Build history of the part. All positions in model axes, mm. A direction names the side the tool comes from. Coordinates: 2 decimals unless noted, no trailing zeros. Loops run counter-clockwise (first coordinate to the right, second up) from the corner with the lowest first, then second, coordinate; pieces in that order, holes last.
(1) Slice it at B-B (z = 6). Give the number of separate pieces and of enclosed holes in the cut face, and give its area (3 significant figures).
(2) Two-plate mould, pull along Y, no slides. Class faces 1 (the face through (229.026, 329.954, 5.916)), 2 (the face through (229.853, 271.613, 5.916)), 3 (the face through (308, 350.56, 6)): pulls with the +Y half, pulls with the -Y half, needs draft (parallel to the pull), parting line crosses it, or undercut.
(3) Slice it at C-C (y = 346). Give the cut face in (x, z).
(4) Wall check: L1, parallel to Y at x = 250, z = 5; L2, parallel to X at y = 274.5, z = 10.5; L3, parallel to X at y = 303, z = 4.5. Give the ranges that are in metal, low to high.
(5) Flat gauge pins, fed straight in: P1, Ø1.5, axis at y = 254.5, z = 5, coming from the +X side; P2, Ø3, axis at y = 349, z = 5.5, coming from the +X side; P3, Ø0.8, axis at y = 348.5, z = 7.5, coming from the -X side; P4, Ø2.5, axis at x = 272.26, y = 244.39, coming from the +Z side. Where does each tip first touch, or does it go through?
(6) Slice it at D-D (x = 326). Give the cut face in (y, z), and give its area (3 significant figures).
(7) Slice it at A-A (x = 308). Give the cut face in (y, z), and give its area (3 significant figures).
(8) Tool access for faces 4 (the face through (309.564, 250.121, 5.916)), 5 (the face through (280, 357.622, 6)): list every direction of +Z, -Z, +X, -X, +Y, -Y with a clear straight run to the whole face (end or side of a thin tool).
from build123d import *

# Parameters (mm, degrees)
ESBO_O1_R                = 2
ESBO_O1_R_2              = 1.5
ESBO_O1_R_3              = 1
ESBO_O1_R_4              = 12
ESBO_O1_W                = 12
ESBO_O1_H                = 2.6
RESSALTO_EXTRUS_O1_DEPTH = 12


with BuildPart() as part:
    # Esboço1 → Ressalto-extrusão1 (new body)
    with BuildSketch(Plane.XY):
        Polygon((312.401923789, 240.878221735), (347.401923789, 301.5), (315, 357.621778265), (245, 357.621778265), (212.598076211, 301.5), (247.598076211, 240.878221735), align=None)
        with Locations((280, 253.378221735)):
            Circle(ESBO_O1_R, mode=Mode.SUBTRACT)
        with Locations((272.260343171, 244.388972359)):
            Circle(ESBO_O1_R_2, mode=Mode.SUBTRACT)
        with Locations((287.760343171, 244.388972359)):
            Circle(ESBO_O1_R_2, mode=Mode.SUBTRACT)
        with Locations((280, 349.621778265)):
            Circle(ESBO_O1_R_3, mode=Mode.SUBTRACT)
        with Locations((237.026279442, 275.189110868)):
            Circle(ESBO_O1_R_3, mode=Mode.SUBTRACT)
        with Locations((322.973720558, 275.189110868)):
            Circle(ESBO_O1_R_3, mode=Mode.SUBTRACT)
        with Locations((278.32399049, 302.032244112)):
            Circle(ESBO_O1_R_4, mode=Mode.SUBTRACT)
        with Locations((251.453146627, 349.186651246)):
            Rectangle(ESBO_O1_W, ESBO_O1_H, mode=Mode.SUBTRACT)
        with Locations((308.5, 349.259600438)):
            Rectangle(ESBO_O1_W, ESBO_O1_H, mode=Mode.SUBTRACT)
        Polygon((332.76851184, 295.516364843), (335.020177889, 294.216364843), (341.020177889, 304.608669688), (338.76851184, 305.908669688), align=None, mode=Mode.SUBTRACT)
        Polygon((310.272092192, 256.543153732), (312.523758242, 255.243153732), (306.520177889, 244.852916827), (304.26851184, 246.152916827), align=None, mode=Mode.SUBTRACT)
        Polygon((255.623234985, 246.090416827), (253.371568935, 244.790416827), (247.371568935, 255.182721672), (249.623234985, 256.482721672), align=None, mode=Mode.SUBTRACT)
        Polygon((227.123234985, 295.453864843), (224.871568935, 294.153864843), (218.871568935, 304.546169688), (221.123234985, 305.846169688), align=None, mode=Mode.SUBTRACT)
    extrude(amount=RESSALTO_EXTRUS_O1_DEPTH)


solid = part.part
Response values:
1. separate pieces: 1
1. enclosed holes: 13
1. area: 11,100 mm2
2. face 1: pulls with the +Y half
2. face 2: pulls with the -Y half
2. face 3: undercut
3. outline: (238.29, 0) - (321.71, 0) - (321.71, 12) - (238.29, 12) - close
4. L1: y = 240.88 to 250.63, 255.83 to 347.89, 350.49 to 357.62
4. L2: x = 228.19 to 236.3, 237.75 to 322.25, 323.7 to 331.81
4. L3: x = 213.46 to 219.76, 222.77 to 266.36, 290.28 to 337.09, 340.09 to 346.54
5. P1: stops at x = 320.7
5. P2: stops at x = 320.84
5. P3: stops at x = 239.5
5. P4: passes through
6. outline: (264.43, 0) - (338.57, 0) - (338.57, 12) - (264.43, 12) - close
6. area: 890 mm2
7. outline: (240.88, 0) - (247.41, 0) - (247.41, 12) - (240.88, 12) - close; (252.61, 0) - (347.96, 0) - (347.96, 12) - (252.61, 12) - close; (350.56, 0) - (357.62, 0) - (357.62, 12) - (350.56, 12) - close
7. area: 1,310 mm2
8. face 4: +Z, -Z
8. face 5: +Z, -Z, +X, -X, +Y
